Input: dimensioned drawing with shaded views. Units: mm. Origin: part minimum x, y, z. A direction names the side the tool comes from. Give positions to 0.01 mm unless a question says otherwise; leave off trailing zeros. Loops run counter-clockwise (first coordinate to the right, second up) from the corner with the lowest first, then second, coordinate; pieces in that order, holes last.
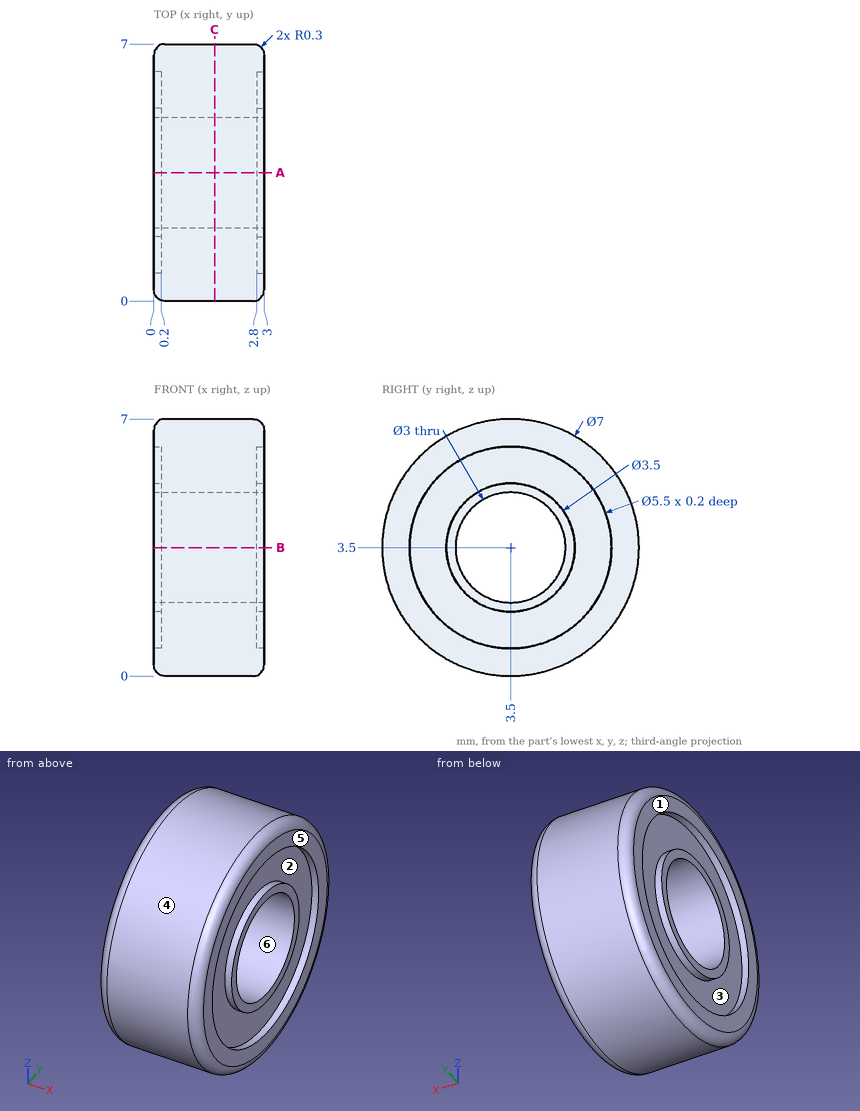
Item 1: Draft query along Y for the marked faces 4, 5 and 6. Return one class per face: +Y half, -Y half, draft (parallel to the pull), parting line (faces both ways), or undercut.
Values follow:
face 4: parting line
face 5: draft
face 6: undercut
Item 2: Section query A-A on y = 3.5. Return loops of the section in (x, z), plus the area to 3 significant figures.
Values follow:
outline: (0, 0.3) arc R0.3 ccw to (0.3, 0) - (2.7, 0) arc R0.3 ccw to (3, 0.3) - (3, 0.75) - (2.8, 0.75) - (2.8, 1.75) - (3, 1.75) - (3, 2) - (0, 2) - (0, 1.75) - (0.2, 1.75) - (0.2, 0.75) - (0, 0.75) - close; (0, 5) - (3, 5) - (3, 5.25) - (2.8, 5.25) - (2.8, 6.25) - (3, 6.25) - (3, 6.7) arc R0.3 ccw to (2.7, 7) - (0.3, 7) arc R0.3 ccw to (0, 6.7) - (0, 6.25) - (0.2, 6.25) - (0.2, 5.25) - (0, 5.25) - close
area: 11.1 mm2
Item 3: Ray query, probe 1 along Z at (x, y) = (1.15, 3.75); probe 2 along X at (y, z) = (4, 5.5). Return the intervals inside material, ascending.
Values follow:
probe 1: z = 0.01 to 2.02, 4.98 to 6.99
probe 2: x = 0.2 to 2.8
Item 4: Set-up query: the marked faces 1, 2 and 3. Return all of +Z, -Z, +X, -X, +Y, -Y with unobstructed straight access to the full face (end or side cutting, diameter ignored); none if empty.
Values follow:
face 1: +Z, -Z, -X, +Y, -Y
face 2: +X
face 3: -X
Item 5: Section query C-C on x = 1.65. Return loops of the section in (y, z).
Values follow:
outline: circle Ø7 at (3.5, 3.5); hole circle Ø3 at (3.5, 3.5)
Item 6: Pin query (flat end, axial travel): pin 1 (1.5 mm diameter, centred on x = 1, y = 1.5, fed in from +Z); pin 2 (2.5 mm diameter, centred on y = 3.5, z = 3.5, fed in from -X). Return the tip coordinate at first contact, or that it passes through.
Values follow:
pin 1: stops at z = 6.77
pin 2: passes through
